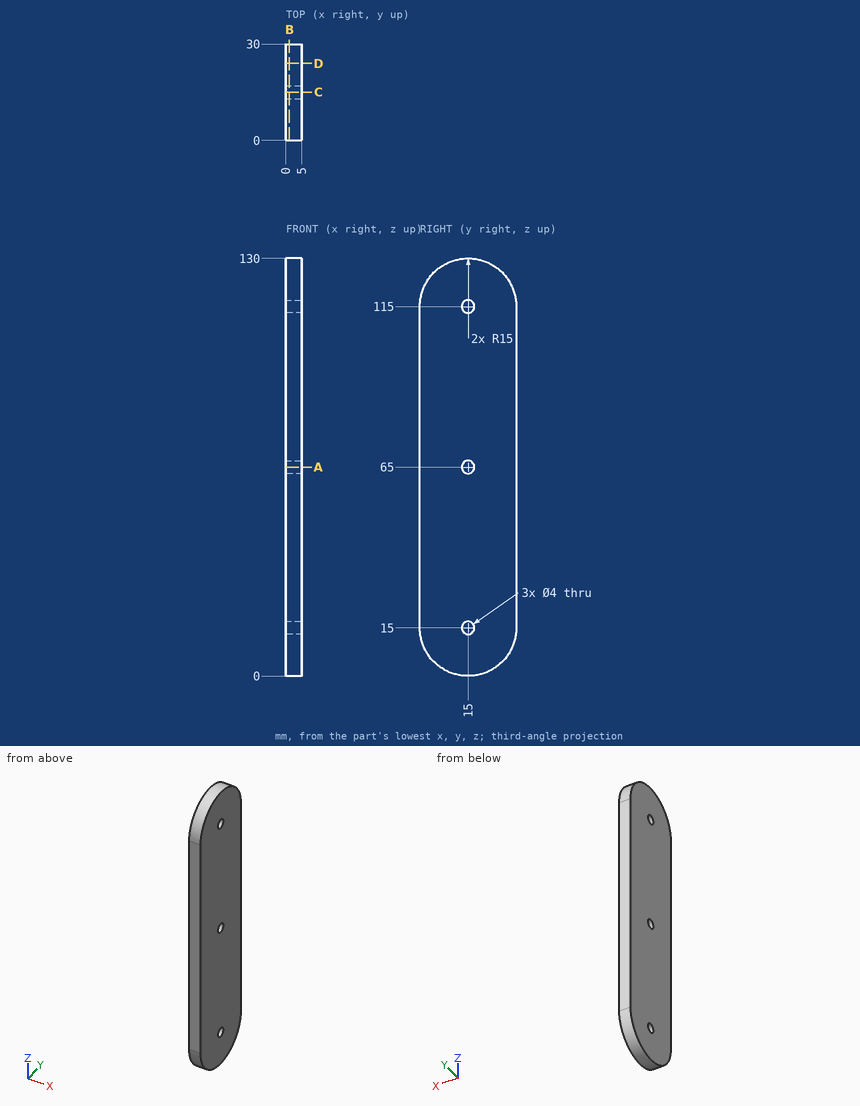
Input: dimensioned drawing with shaded views. Units: mm. Origin: part minimum x, y, z. Give positions to 0.01 mm unless a question says otherwise; leave off trailing zeros. Write each loop counter-clockwise with the first axis right and the second up, starting at its lowest first coordinate (ties: lowest second). Pieces come first, ordered by that corner, then holes.
1. Section query B-B (x = 1.1). Return the cut outline in (y, z), then the cut area to 3 significant figures.
2. Section query D-D (y = 24). Return the cut outline in (x, z).
3. Material intervals for line 1 along Y through (x, z) = (3.1, 115); line 2 along Z through (x, y) = (1.6, 3.5); line 3 along Z through (x, y) = (0.85, 11.5), sorted ascending.
4. First-contact query: pin 1 (3 mm diameter, centred on x = 3, y = 23, fed in from +Z). Flat tip, straight axial feed; report the tip coordinate or a pass-through.
5. Section query C-C (y = 15). Return the cut outline in (x, z).
6. Section query A-A (z = 65). Return the cut outline in (x, y), then the cut area to 3 significant figures.
Output values:
1. outline: (0, 15) arc R15 ccw to (30, 15) - (30, 115) arc R15 ccw to (0, 115) - close; hole circle Ø4 at (15, 15); hole circle Ø4 at (15, 65); hole circle Ø4 at (15, 115)
1. area: 3,670 mm2
2. outline: (0, 3) - (5, 3) - (5, 127) - (0, 127) - close
3. line 1: y = 0 to 13, 17 to 30
3. line 2: z = 5.37 to 124.63
3. line 3: z = 0.41 to 129.59
4. pin 1: stops at z = 128.52
5. outline: (0, 0) - (5, 0) - (5, 13) - (0, 13) - close; (0, 17) - (5, 17) - (5, 63) - (0, 63) - close; (0, 67) - (5, 67) - (5, 113) - (0, 113) - close; (0, 117) - (5, 117) - (5, 130) - (0, 130) - close
6. outline: (0, 0) - (5, 0) - (5, 13) - (0, 13) - close; (0, 17) - (5, 17) - (5, 30) - (0, 30) - close
6. area: 130 mm2
